Can you work these out from the drawing? Everything is in mm from the part's minimum corner. A direction names the side the tool comes from. Round coordinates to 2 decimals unless told otherwise and drop trailing zeros. Order: outer loops, then holes, each group sorted by start corner. A loop starts at its lowest first (then second) coordinate and runs counter-clockwise, first axis right, second up. Notation, with made-up numbers: (-23.5, 4) - (29.5, 4) arc R17 cw to (29.5, 37) - close; hole circle Ø5 at (-34.5, 29.25). An arc over 180 degrees is marked (long way). Write item = value, one per line.
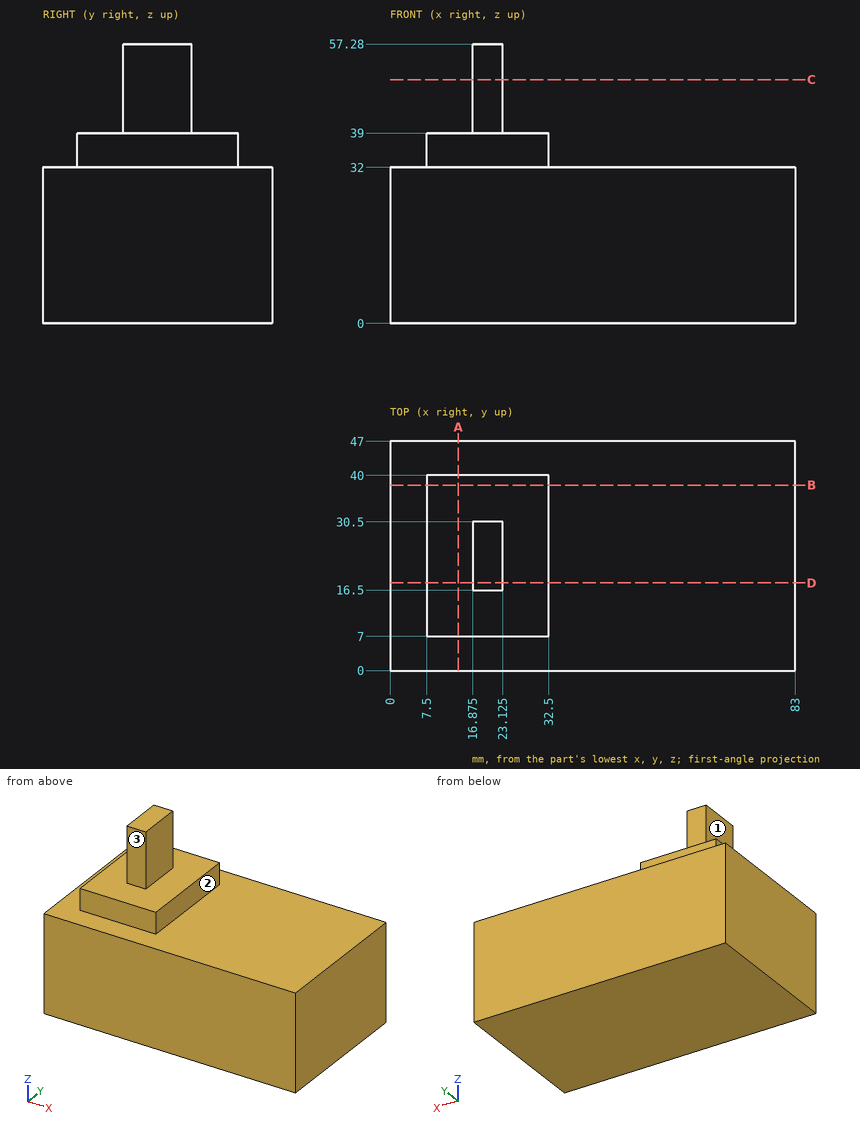
(1) On a 3-axis mill with a long thin cutter (end or side, diameter ignored), from which of +Z, -Z, +X, -X, +Y, -Y can I reach the whole of each face in a straight line? I mean the marked faces 1, 2 and 3. Say none if no direction works.
Computed:
face_1 = +Z, -X, +Y, -Y
face_2 = +Z, +X, +Y, -Y
face_3 = +Z, +X, -X, -Y
(2) If we section it at A-A (x = 14): Write out the boundary of the cut face in (y, z), plus the area to 4 significant figures.
Computed:
outline = (0, 0) - (47, 0) - (47, 32) - (40, 32) - (40, 39) - (7, 39) - (7, 32) - (0, 32) - close
area = 1,735 mm^2
(3) If I drill on line 1 (Z direction, x = 30.5, y = 15); line 2 (Z direction, x = 4, y = 35); line 3 (X direction, y = 22.5, z = 48) (3 decimals), over which ranges is the centre line in solid material (lowest first)? Write a range as from..to.
Computed:
line_1 = 0..39
line_2 = 0..32
line_3 = 16.875..23.125
(4) Will these pins go through, and if not, where does the flat tip stop? P1, Ø15.5, axis at y = 20, z = 49, coming from the +X side (3 decimals); P2, Ø15.5, axis at y = 25, z = 46.5, coming from the -X side; P3, Ø1, axis at x = 15, y = 34, coming from the +Z side; P4, Ø1, axis at x = 10, y = 8.5, coming from the -Z side.
Computed:
P1 = 23.125
P2 = 7.5
P3 = 39
P4 = 0
(5) If we section it at B-B (y = 38): Write out the boundary of the cut face in (x, z), plus the area to 3 significant figures.
Computed:
outline = (0, 0) - (83, 0) - (83, 32) - (32.5, 32) - (32.5, 39) - (7.5, 39) - (7.5, 32) - (0, 32) - close
area = 2,830 mm^2
(6) If we section it at D-D (y = 18): Write out the boundary of the cut face in (x, z) (3 decimals).
Computed:
outline = (0, 0) - (83, 0) - (83, 32) - (32.5, 32) - (32.5, 39) - (23.125, 39) - (23.125, 57.28) - (16.875, 57.28) - (16.875, 39) - (7.5, 39) - (7.5, 32) - (0, 32) - close
(7) If we section it at C-C (z = 50): Write out the boundary of the cut face in (x, y) (3 decimals).
Computed:
outline = (16.875, 16.5) - (23.125, 16.5) - (23.125, 30.5) - (16.875, 30.5) - close
